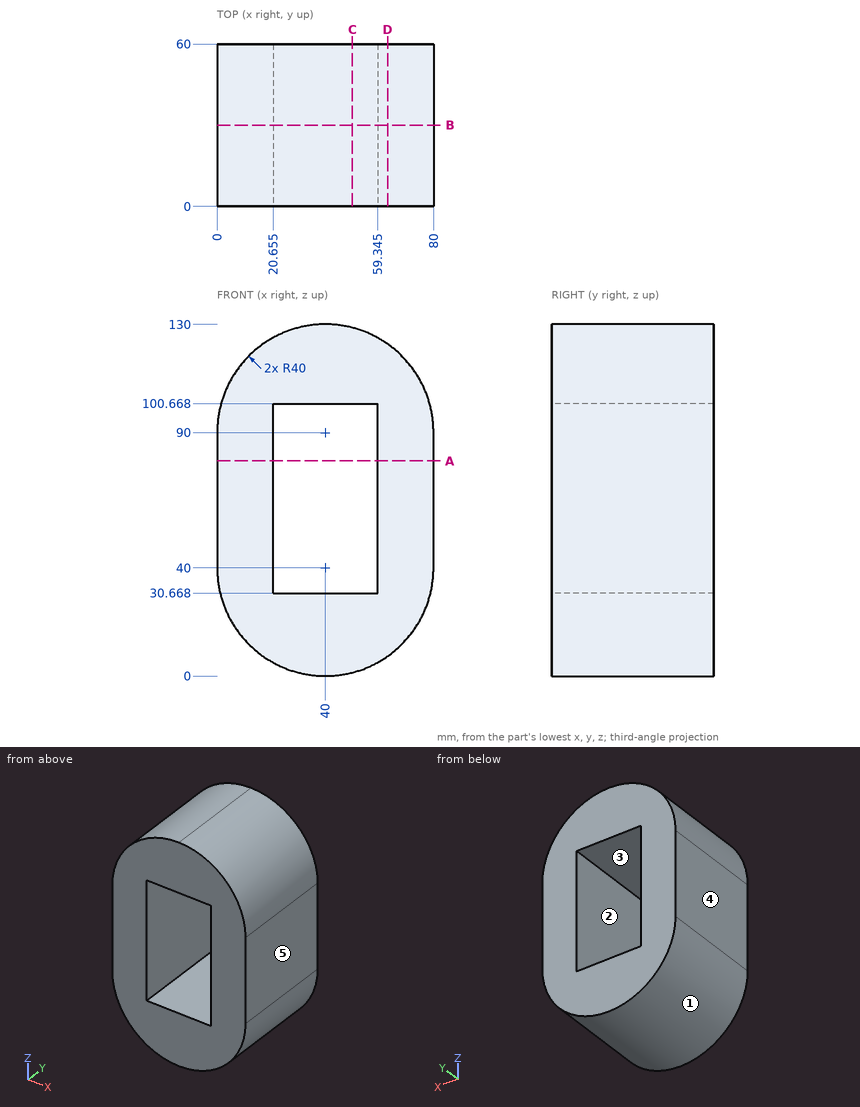
Verification items for this drawing (mm, ordinates from the low corner). A direction names the side the tool comes from. Round coordinates to 2 decimals unless told otherwise and drop trailing zeros. Write each loop counter-clockwise with the first axis right and the second up, starting at its lowest first coordinate (ties: lowest second). Pieces come first, ordered by that corner, then holes. Notation, with made-up numbers: (88, 72) - (146, 72) arc R12 cw to (146, 95) - close; hole circle Ø3 at (33, 68.25). An arc over 180 degrees is marked (long way). One line per item, written item: value.
1. Scan lines: L1, parallel to X at y = 4, z = 67 (1 decimal); L2, parallel to X at y = 57, z = 34 (1 decimal); L3, parallel to Z at x = 32.5, y = 25.5. Record each from-to range of solid material in increasing order.
The answers:
L1: x = 0 to 20.7, 59.3 to 80
L2: x = 0.5 to 20.7, 59.3 to 79.5
L3: z = 0.71 to 30.67, 100.67 to 129.29
2. Mould release check, pull along X, two halves, no side actions. Record for the marked faces 3, 4 and 5: released by +X, released by -X, zero draft, split by the parting line, or undercut.
The answers:
face 3: undercut
face 4: released by -X
face 5: released by +X
3. Depth check by flat-ended pin: pin 1 Ø2 at (y, z) = (46.5, 100.5) entering from -X (1 decimal). Enter the tip coordinate at first touch or a pass-through.
The answers:
pin 1: stops at x = 1.1
4. Cross-section at C-C on x = 50. Record the boundary of the cut face in (y, z).
The answers:
outline: (0, 1.27) - (60, 1.27) - (60, 30.67) - (0, 30.67) - close; (0, 100.67) - (60, 100.67) - (60, 128.73) - (0, 128.73) - close
5. Cross-section at B-B on y = 30. Record the boundary of the cut face in (x, z) (1 decimal).
The answers:
outline: (0, 40) arc R40 ccw to (80, 40) - (80, 90) arc R40 ccw to (40, 130) arc R40 ccw to (0, 90) - close; hole (20.7, 30.7) - (59.3, 30.7) - (59.3, 100.7) - (20.7, 100.7) - close
6. Cross-section at A-A on z = 79.5. Record the boundary of the cut face in (x, y) (1 decimal), and give its area (3 significant figures).
The answers:
outline: (0, 0) - (20.7, 0) - (20.7, 60) - (0, 60) - close; (59.3, 0) - (80, 0) - (80, 60) - (59.3, 60) - close
area: 2,480 mm^2
7. Set-up check for the marked faces 1 and 2: record each of +Z, -Z, +X, -X, +Y, -Y from which the full face is reachable in a straight line by a thin tool's end or side.
The answers:
face 1: -Z, +Y, -Y
face 2: +Y, -Y
8. Cross-section at D-D on x = 63. Record the boundary of the cut face in (y, z).
The answers:
outline: (0, 7.27) - (60, 7.27) - (60, 122.73) - (0, 122.73) - close
